```python
from build123d import *

# Parameters (mm, degrees)
BASE_FLANGE1_DEPTH      = 130
SKETCH6_R               = 3
CUT_EXTRUDE1_DEPTH      = 10
HEM1_DEPTH              = 130
CUT_EXTRUDE2_DEPTH      = 169.205231785
CUT_EXTRUDE2_DEPTH_BACK = 169.205231785
SKETCH7_R               = 13
SKETCH7_R_2             = 7.5
EDGE_FLANGE1_DEPTH      = 130
CUT_EXTRUDE3_DEPTH      = 47


# Read off the part's stored shape, not the designer's step: Hem1
# Sheet-metal steps are written as plain solids
with BuildPart() as part:
    # Sketch1 → Base-Flange1 (new body)
    with BuildSketch(Plane.XY):
        with BuildLine():
            Line((0, 100), (0, 4))
            ThreePointArc((0, 4), (-1.171572875, 1.171572875), (-4, 0))
            Line((-4, 0), (-30, 0))
            Line((-30, 0), (-30, 2))
            Line((-30, 2), (-4, 2))
            ThreePointArc((-4, 2), (-2.585786438, 2.585786438), (-2, 4))
            Line((-2, 4), (-2, 100))
            Line((-2, 100), (0, 100))
        make_face()
    extrude(amount=BASE_FLANGE1_DEPTH)

    # Sketch6 → Cut-Extrude1 (cut)
    with BuildSketch(Plane(origin=(0, 2, 0), x_dir=(1, 0, 0), z_dir=(0, 1, 0))):
        with Locations(Location((-15, -15, 0), (0, 0, 270))):
            Circle(SKETCH6_R)
        with Locations(Location((-15, -115, 0), (0, 0, 270))):
            Circle(SKETCH6_R)
    extrude(amount=-CUT_EXTRUDE1_DEPTH, mode=Mode.SUBTRACT)

    # Hem1 outline → Hem1 (add)
    with BuildSketch(Plane.XY):
        with BuildLine():
            Line((2, 6), (4, 6))
            Line((4, 6), (4, 100))
            ThreePointArc((4, 100), (1, 103), (-2, 100))
            Line((-2, 100), (0, 100))
            ThreePointArc((0, 100), (1, 101), (2, 100))
            Line((2, 100), (2, 6))
        make_face()
    extrude(amount=HEM1_DEPTH)

    # Sketch7 → Cut-Extrude2 (cut, two sides: drawn at the far end of the back side and taken through both)
    with BuildSketch(Plane.ZY.offset(2).offset(-CUT_EXTRUDE2_DEPTH_BACK)):
        with Locations(Location((65, 84.5, 0), (0, 0, 270))):
            Circle(SKETCH7_R)
        with Locations(Location((15, 25.347000811, 0), (0, 0, 270))):
            Circle(SKETCH7_R_2)
        with BuildLine():
            Line((72.5, 29.347000811), (117.5, 29.347000811))
            ThreePointArc((117.5, 29.347000811), (121.5, 25.347000811), (117.5, 21.347000811))
            Line((117.5, 21.347000811), (72.5, 21.347000811))
            ThreePointArc((72.5, 21.347000811), (68.5, 25.347000811), (72.5, 29.347000811))
        make_face()
        with BuildLine():
            Line((72.5, 36.847000811), (117.5, 36.847000811))
            ThreePointArc((117.5, 36.847000811), (119, 35.347000811), (117.5, 33.847000811))
            Line((117.5, 33.847000811), (72.5, 33.847000811))
            ThreePointArc((72.5, 33.847000811), (71, 35.347000811), (72.5, 36.847000811))
        make_face()
        with BuildLine():
            Line((72.5, 13.847000811), (117.5, 13.847000811))
            ThreePointArc((117.5, 13.847000811), (119, 15.347000811), (117.5, 16.847000811))
            Line((117.5, 16.847000811), (72.5, 16.847000811))
            ThreePointArc((72.5, 16.847000811), (71, 15.347000811), (72.5, 13.847000811))
        make_face()
    extrude(amount=CUT_EXTRUDE2_DEPTH + CUT_EXTRUDE2_DEPTH_BACK, mode=Mode.SUBTRACT)

    # Edge-Flange1 section (across the edge) → Edge-Flange1 (add)
    with BuildSketch(Plane(origin=(-32, 2, 0), x_dir=(1, 0, 0), z_dir=(0, 0, 1))):
        with BuildLine():
            Line((-2, 2), (-2, 48))
            Line((-2, 48), (0, 48))
            Line((0, 48), (0, 2))
            ThreePointArc((0, 2), (0.585786438, 0.585786438), (2, 0))
            Line((2, 0), (2, -2))
            ThreePointArc((2, -2), (-0.828427125, -0.828427125), (-2, 2))
        make_face()
    extrude(amount=EDGE_FLANGE1_DEPTH)

    # Sketch7<2> → Cut-Extrude3 (cut)
    with BuildSketch(Plane.ZY.offset(2)):
        with BuildLine():
            Line((72.5, 33.847000811), (117.5, 33.847000811))
            ThreePointArc((117.5, 33.847000811), (119, 35.347000811), (117.5, 36.847000811))
            Line((117.5, 36.847000811), (72.5, 36.847000811))
            ThreePointArc((72.5, 36.847000811), (71, 35.347000811), (72.5, 33.847000811))
        make_face()
        with BuildLine():
            Line((72.5, 21.347000811), (117.5, 21.347000811))
            ThreePointArc((117.5, 21.347000811), (121.5, 25.347000811), (117.5, 29.347000811))
            Line((117.5, 29.347000811), (72.5, 29.347000811))
            ThreePointArc((72.5, 29.347000811), (68.5, 25.347000811), (72.5, 21.347000811))
        make_face()
        with BuildLine():
            ThreePointArc((117.5, 16.847000811), (119, 15.347000811), (117.5, 13.847000811))
            Line((117.5, 13.847000811), (72.5, 13.847000811))
            ThreePointArc((72.5, 13.847000811), (71, 15.347000811), (72.5, 16.847000811))
            Line((72.5, 16.847000811), (117.5, 16.847000811))
        make_face()
    extrude(amount=CUT_EXTRUDE3_DEPTH, mode=Mode.SUBTRACT)


solid = part.part
```
The listing builds one solid part. Answer for the finished solid, in the listing's coordinates (mm). A direction names the side the tool comes from. Give positions to 0.01 mm unless a question says otherwise; leave off trailing zeros. Order: outer loops, then holes, each group sorted by start corner. A loop starts at its lowest first (then second) coordinate and runs counter-clockwise, first axis right, second up. Notation, with made-up numbers: (7.5, 57.25) -> (13.5, 57.25) arc R17 ccw to (13.5, 90.25) -> close; hole circle Ø7 at (28.5, 12). An arc over 180 degrees is marked (long way). Write each question's results on one line, items separated by ' | '.
Q1. The part is cut by section D-D, the plane z = 100. State how many separate pieces and enclosed holes the cut face has, and give its area (3 significant figures).
Checked values:
separate pieces: 10 | enclosed holes: 0 | area: 471 mm^2
Q2. The part is cut by section B-B, the plane y = 84.5. Give the vertices of the cut face in (x, z), and give its area (3 significant figures).
Checked values:
outline: (-2, 0) -> (0, 0) -> (0, 52) -> (-2, 52) -> close; (-2, 78) -> (0, 78) -> (0, 130) -> (-2, 130) -> close; (2, 0) -> (4, 0) -> (4, 52) -> (2, 52) -> close; (2, 78) -> (4, 78) -> (4, 130) -> (2, 130) -> close | area: 416 mm^2
Q3. The part is cut by section A-A, the plane z = 15. Give the vertices of the cut face in (x, y).
Checked values:
outline: (-34, 4) arc R4 ccw to (-30, 0) -> (-18, 0) -> (-18, 2) -> (-30, 2) arc R2 cw to (-32, 4) -> (-32, 50) -> (-34, 50) -> close; (-12, 0) -> (-4, 0) arc R4 ccw to (0, 4) -> (0, 17.85) -> (-2, 17.85) -> (-2, 4) arc R2 cw to (-4, 2) -> (-12, 2) -> close; (-2, 32.85) -> (0, 32.85) -> (0, 100) arc R1 cw to (2, 100) -> (2, 32.85) -> (4, 32.85) -> (4, 100) arc R3 ccw to (-2, 100) -> close; (2, 6) -> (4, 6) -> (4, 17.85) -> (2, 17.85) -> close
Q4. Which of the six approach directions +Z, -Z, +X, -X, +Y, -Y give full straight-line access (tool end or side, diameter ignored) to faces 4 (the face through (-2, 51, 64)), 5 (the face through (-1, 25.3, 68.5)), 6 (the face through (0, 53, 64))?
Checked values:
face 4: +Z, -Z, +Y | face 5: +X, -X | face 6: +Z, -Z, -Y
Q5. Determine the mould class of faces 1 (the face through (-17, 2, 64)), 2 (the face through (3, 25.4, 121.5)), 3 (the face through (-34, 27, 64)) for opening direction X: pulls with the +X half, pulls with the -X half, needs draft (parallel to the pull), parting line crosses it, or undercut.
Checked values:
face 1: undercut | face 2: needs draft | face 3: pulls with the -X half
Q6. The part is cut by section C-C, the plane x = -15. Give the vertices of the cut face in (y, z).
Checked values:
outline: (0, 0) -> (2, 0) -> (2, 12) -> (0, 12) -> close; (0, 18) -> (2, 18) -> (2, 112) -> (0, 112) -> close; (0, 118) -> (2, 118) -> (2, 130) -> (0, 130) -> close
Q7. Straight lines are drawn through the part: probe 1 along X at (y, z) = (39, 28); probe 2 along X at (y, z) = (50.5, 23); probe 3 along Z at (x, y) = (3.1, 84.5). For each, find the intervals that lie inside material, in ascending order. Write a range as from..to.
Checked values:
probe 1: x = -34..-32, -2..0, 2..4 | probe 2: x = -2..0, 2..4 | probe 3: z = 0..52, 78..130
Q8. Each of these flat-tipped pins is pushed along its axis until it touches: P1, Ø1, axis at x = -33, z = 104.5, coming from the -Y side; P2, Ø0.6, axis at x = 3.5, z = 85, coming from the -Y side; P3, Ø1.6, axis at x = 3, z = 104, coming from the +Y side; P4, Ø10, axis at x = -26, y = 20, coming from the +Z side. Where does it stop, or does it pass through?
Checked values:
P1: stops at y = 0.88 | P2: stops at y = 6 | P3: stops at y = 102.75 | P4: passes through
